Source: CAD feature listing. Evaluate the final solid. Frame: model axes, mm. Face numbers are marked on the shaded views. Coordinates: 2 decimals unless noted, no trailing zeros. Write each loop counter-clockwise with the first axis right and the second up, starting at its lowest first coordinate (ties: lowest second). Pieces come first, ordered by that corner, then holes. Notation, with made-up numbers: (10, 40) - (18, 40) arc R24 ccw to (18, 63) - close; hole circle Ø6 at (-35, 70.25). An arc over 180 degrees is marked (long way). One line per question, with ' | ' between items.
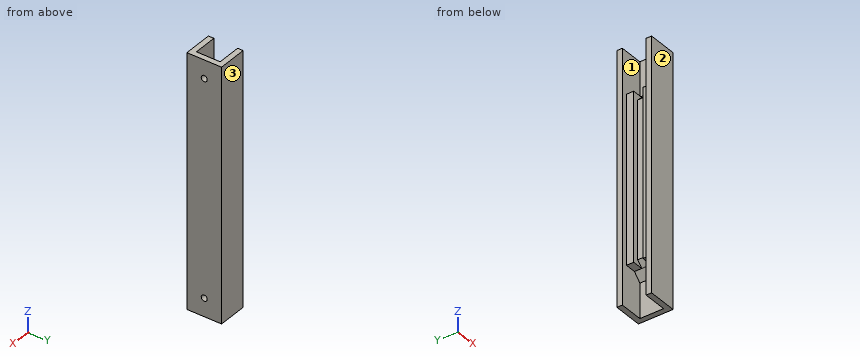
from build123d import *

# Parameters (mm, degrees)
SKETCH_1_W          = 19
SKETCH_1_H          = 19
SKETCH_1_W_2        = 13
SKETCH_1_H_2        = 13
EXTRUDE_1_DEPTH     = 137.7
SKETCH_2_R          = 1.65
CUT_EXTRUDE_1_DEPTH = 30
SKETCH_3_W          = 184.332972064
SKETCH_3_H          = 39.863215684
CUT_EXTRUDE_2_DEPTH = 3
SKETCH_4_W          = 5
SKETCH_4_H          = 13
EXTRUDE_1_2_DEPTH   = 10
SKETCH_5_W          = 81.7
SKETCH_5_H          = 5
EXTRUDE_2_DEPTH     = 10
SKETCH_6_W          = 91.7
SKETCH_6_H          = 13
EXTRUDE_3_DEPTH     = 10
SKETCH_8_W          = 91.7
SKETCH_8_H          = 5
CUT_EXTRUDE_3_DEPTH = 3
CHAMFER_1_SIZE      = 3
CHAMFER_2_SIZE      = 4


with BuildPart() as part:
    # 草图1 → Extrude 1 (new body)
    with BuildSketch(Plane.XY):
        with Locations((6.5, 6.5)):
            Rectangle(SKETCH_1_W, SKETCH_1_H)
        with Locations((6.5, 6.5)):
            Rectangle(SKETCH_1_W_2, SKETCH_1_H_2, mode=Mode.SUBTRACT)
    extrude(amount=EXTRUDE_1_DEPTH)

    # 草图2 → 切除-拉伸1 (cut)
    with BuildSketch(Plane.ZY.offset(3)):
        with Locations((10, 6.5)):
            Circle(SKETCH_2_R)
        with Locations((127.7, 6.5)):
            Circle(SKETCH_2_R)
    extrude(amount=-CUT_EXTRUDE_1_DEPTH, mode=Mode.SUBTRACT)

    # 草图3 → 切除-拉伸2 (cut)
    with BuildSketch(Plane.ZY.offset(3)):
        with Locations((86.871134348, 3.380889782)):
            Rectangle(SKETCH_3_W, SKETCH_3_H)
    extrude(amount=-CUT_EXTRUDE_2_DEPTH, mode=Mode.SUBTRACT)

    # 草图4 → Extrude 1 2 (add)
    with BuildSketch(Plane.ZY.offset(-13)):
        with Locations((25.5, 6.5)):
            Rectangle(SKETCH_4_W, SKETCH_4_H)
        with Locations((112.2, 6.5)):
            Rectangle(SKETCH_4_W, SKETCH_4_H)
    extrude(amount=EXTRUDE_1_2_DEPTH)

    # 草图5 → 凸台-拉伸2 (add)
    with BuildSketch(Plane.ZY.offset(-13)):
        with Locations((68.85, 6.5)):
            Rectangle(SKETCH_5_W, SKETCH_5_H)
    extrude(amount=EXTRUDE_2_DEPTH)

    # 草图6 → 凸台-拉伸3 (add)
    with BuildSketch(Plane.ZY.offset(-13)):
        with Locations((68.85, 6.5)):
            Rectangle(SKETCH_6_W, SKETCH_6_H)
    extrude(amount=EXTRUDE_3_DEPTH)

    # 草图8 → 切除-拉伸3 (cut)
    with BuildSketch(Plane.ZY.offset(-3)):
        with Locations((68.85, 6.5)):
            Rectangle(SKETCH_8_W, SKETCH_8_H)
    extrude(amount=-CUT_EXTRUDE_3_DEPTH, mode=Mode.SUBTRACT)

    # 倒角1
    chamfer_1_edges = [part.edges().sort_by_distance(p)[0] for p in [
        (6, 6.5, 23),
        (6, 6.5, 114.7),
    ]]
    chamfer(chamfer_1_edges, length=CHAMFER_1_SIZE)

    # 倒角2
    chamfer_2_edges = [part.edges().sort_by_distance(p)[0] for p in [
        (13, 6.5, 23),
        (13, 6.5, 114.7),
    ]]
    chamfer(chamfer_2_edges, length=CHAMFER_2_SIZE - 0.0001)  # a hair under: the kernel refuses the full size


solid = part.part
Item 1: Cut plane A-A on y = 6.5. State how many separate pieces and enclosed holes the cut face has, and give its area (3 significant figures).
Check sheet entries:
separate pieces: 3 | enclosed holes: 0 | area: 1,040 mm²
Item 2: Ray query, line 1 along Y through (x, z) = (13.85, 127.7); line 2 along Y through (x, z) = (10.25, 21.5); line 3 along Z through (x, y) = (13.75, 5). Return the intervals inside material, ascending. Write a range as [from, to].
Check sheet entries:
line 1: [-3, 4.85], [8.15, 16] | line 2: [-3, 0], [13, 16] | line 3: [0, 9.31], [10.69, 127.01], [128.39, 137.7]
Item 3: Mould query, pull axis Y, two halves, no side actions, for the marked faces 1, 2 and 3. Classes: pulls with the +Y half, pulls with the -Y half, needs draft (parallel to the pull), parting line crosses it, or undercut.
Check sheet entries:
face 1: undercut | face 2: pulls with the -Y half | face 3: pulls with the +Y half
Item 4: Pin query (flat end, axial travel): pin 1 Ø1 at (x, y) = (5, 11) entering from +Z; pin 2 Ø3 at (x, y) = (6.5, 8.5) entering from -Z; pin 3 Ø1.5 at (y, z) = (5.5, 50) entering from -X. Return the tip coordinate at first contact, or that it passes through.
Check sheet entries:
pin 1: z = 114.7 | pin 2: z = 23 | pin 3: x = 6
Item 5: Cut plane C-C on z = 127.7. Return loops of the section in (x, y).
Check sheet entries:
outline: (0, -3) - (16, -3) - (16, 4.85) - (13, 4.85) - (13, 0) - (0, 0) - close; (0, 13) - (13, 13) - (13, 8.15) - (16, 8.15) - (16, 16) - (0, 16) - close
Item 6: Cut plane D-D on z = 77. Return loops of the section in (x, y), and give its area (3 significant figures).
Check sheet entries:
outline: (0, -3) - (16, -3) - (16, 16) - (0, 16) - (0, 13) - (3, 13) - (3, 9) - (6, 9) - (6, 4) - (3, 4) - (3, 0) - (0, 0) - close | area: 250 mm²
Item 7: Cut plane B-B on x = 1.5. Return loops of the section in (y, z).
Check sheet entries:
outline: (-3, 0) - (0, 0) - (0, 137.7) - (-3, 137.7) - close; (13, 0) - (16, 0) - (16, 137.7) - (13, 137.7) - close
